from build123d import *

# Parameters (mm, degrees)
BOSS_EXTRUDE1_DEPTH  = 90
SKETCH2_W            = 30
SKETCH2_H            = 40
CUT_EXTRUDE1_DEPTH   = 90
SKETCH3_W            = 20
SKETCH3_H            = 20
CUT_EXTRUDE2_DEPTH   = 90
SKETCH4_W            = 80
SKETCH4_H            = 20
CUT_EXTRUDE3_DEPTH   = 90
SKETCH5_W            = 30
SKETCH5_H            = 30
CUT_EXTRUDE4_DEPTH   = 90
CUT_EXTRUDE6_DEPTH   = 40
BOSS_EXTRUDE6_DEPTH  = 30
CUT_EXTRUDE7_DEPTH   = 20
SKETCH12_W           = 10
SKETCH12_H           = 30
CUT_EXTRUDE8_DEPTH   = 20
SKETCH13_W           = 20
SKETCH13_H           = 30
CUT_EXTRUDE9_DEPTH   = 20
SKETCH14_W           = 21.421822341
SKETCH14_H           = 40
BOSS_EXTRUDE7_DEPTH  = 10
SKETCH16_W           = 20
SKETCH16_H           = 60
BOSS_EXTRUDE8_DEPTH  = 30
SKETCH17_W           = 30
SKETCH17_H           = 30
CUT_EXTRUDE10_DEPTH  = 20
SKETCH18_W           = 90
SKETCH18_H           = 30
BOSS_EXTRUDE9_DEPTH  = 10
SKETCH19_W           = 90
SKETCH19_H           = 20
BOSS_EXTRUDE10_DEPTH = 20
SKETCH21_W           = 10.0001
SKETCH21_H           = 30
BOSS_EXTRUDE13_DEPTH = 30
SKETCH22_W           = 10
SKETCH22_H           = 30
CUT_EXTRUDE13_DEPTH  = 29.999
SKETCH23_W           = 30
SKETCH23_H           = 29.999
CUT_EXTRUDE14_DEPTH  = 1
SKETCH24_W           = 10.0001
SKETCH24_H           = 30
CUT_EXTRUDE15_DEPTH  = 1
SKETCH25_W           = 10
SKETCH25_H           = 30
CUT_EXTRUDE16_DEPTH  = 10
SKETCH27_W           = 10
SKETCH27_H           = 10
CUT_EXTRUDE18_DEPTH  = 30
SKETCH30_W           = 20
SKETCH30_H           = 20
BOSS_EXTRUDE16_DEPTH = 30
SKETCH31_W           = 30
SKETCH31_H           = 20
BOSS_EXTRUDE17_DEPTH = 10


with BuildPart() as part:
    # Sketch1 → Boss-Extrude1 (new body)
    with BuildSketch(Plane.XY):
        with BuildLine():
            ThreePointArc((0, -40), (40, 0), (0, 40))
            Line((0, 40), (0, 20))
            ThreePointArc((0, 20), (14.142135624, 14.142135624), (20, 0))
            ThreePointArc((20, 0), (0, -20), (-20, 0))
            Line((-20, 0), (-40, 0))
            ThreePointArc((-40, 0), (-28.284271247, -28.284271247), (0, -40))
        make_face()
        with BuildLine():
            Line((70, 40), (0, 40))
            ThreePointArc((0, 40), (40, 0), (0, -40))
            Line((0, -40), (70, -40))
            Line((70, -40), (70, 40))
        make_face()
    extrude(amount=BOSS_EXTRUDE1_DEPTH)

    # Sketch2 → Cut-Extrude1 (cut)
    with BuildSketch(Plane.XY.offset(90)):
        with Locations((55, 0)):
            Rectangle(SKETCH2_W, SKETCH2_H)
    extrude(amount=-CUT_EXTRUDE1_DEPTH, mode=Mode.SUBTRACT)

    # Sketch3 → Cut-Extrude2 (cut)
    with BuildSketch(Plane.XY.offset(90)):
        with Locations((60, 30)):
            Rectangle(SKETCH3_W, SKETCH3_H)
    extrude(amount=-CUT_EXTRUDE2_DEPTH, mode=Mode.SUBTRACT)

    # Sketch4 → Cut-Extrude3 (cut)
    with BuildSketch(Plane(origin=(0, -40, 0), x_dir=(1, 0, 0), z_dir=(0, 1, 0))):
        with Locations((0, -80)):
            Rectangle(SKETCH4_W, SKETCH4_H)
    extrude(amount=CUT_EXTRUDE3_DEPTH, mode=Mode.SUBTRACT)

    # Sketch5 → Cut-Extrude4 (cut)
    with BuildSketch(Plane(origin=(0, 0, 0), x_dir=(0, 0, -1), z_dir=(1, 0, 0))):
        with Locations((-85, 25)):
            Rectangle(SKETCH5_W, SKETCH5_H)
    extrude(amount=CUT_EXTRUDE4_DEPTH, mode=Mode.SUBTRACT)

    # Sketch7 → Cut-Extrude6 (cut)
    with BuildSketch(Plane.XY.offset(70)):
        with BuildLine():
            Line((20, 0), (40, 0))
            Line((40, 0), (40, 40))
            Line((40, 40), (0, 40))
            Line((0, 40), (0, 20))
            ThreePointArc((0, 20), (14.142135624, 14.142135624), (20, 0))
        make_face()
    extrude(amount=-CUT_EXTRUDE6_DEPTH, mode=Mode.SUBTRACT)

    # Sketch10 → Boss-Extrude6 (add)
    with BuildSketch(Plane(origin=(70, 0, 0), x_dir=(0, 0, -1), z_dir=(1, 0, 0))):
        Polygon((-70, 20), (-70, 10), (-90, 10), (-90, -20), (-37.089362558, -20), (-21.421822341, -20), (-21.421822341, 20), align=None)
    extrude(amount=-BOSS_EXTRUDE6_DEPTH)

    # Sketch11 → Cut-Extrude7 (cut)
    with BuildSketch(Plane(origin=(70, 0, 0), x_dir=(0, 0, -1), z_dir=(1, 0, 0))):
        Polygon((-21.421822341, -20), (-70, -20), (-70, 10), (-70, 20), (-21.421822341, 20), align=None)
    extrude(amount=-CUT_EXTRUDE7_DEPTH, mode=Mode.SUBTRACT)

    # Sketch12 → Cut-Extrude8 (cut)
    with BuildSketch(Plane(origin=(50, 0, 0), x_dir=(0, 0, -1), z_dir=(1, 0, 0))):
        with Locations((-65, 25)):
            Rectangle(SKETCH12_W, SKETCH12_H)
    extrude(amount=-CUT_EXTRUDE8_DEPTH, mode=Mode.SUBTRACT)

    # Sketch13 → Cut-Extrude9 (cut)
    with BuildSketch(Plane(origin=(0, 0, 70), x_dir=(-1, 0, 0), z_dir=(0, 0, -1))):
        with Locations((-60, -5)):
            Rectangle(SKETCH13_W, SKETCH13_H)
    extrude(amount=-CUT_EXTRUDE9_DEPTH, mode=Mode.SUBTRACT)

    # Sketch14 → Boss-Extrude7 (add)
    with BuildSketch(Plane(origin=(40, 0, 0), x_dir=(0, 0, -1), z_dir=(1, 0, 0))):
        with Locations((-10.710911171, 0)):
            Rectangle(SKETCH14_W, SKETCH14_H)
    extrude(amount=BOSS_EXTRUDE7_DEPTH)

    # Sketch16 → Boss-Extrude8 (add)
    with BuildSketch(Plane(origin=(0, 40, 0), x_dir=(1, 0, 0), z_dir=(0, 1, 0))):
        with Locations((60, -30)):
            Rectangle(SKETCH16_W, SKETCH16_H)
    extrude(amount=-BOSS_EXTRUDE8_DEPTH)

    # Sketch17 → Cut-Extrude10 (cut)
    with BuildSketch(Plane(origin=(70, 0, 0), x_dir=(0, 0, -1), z_dir=(1, 0, 0))):
        with Locations((-15, 25)):
            Rectangle(SKETCH17_W, SKETCH17_H)
    extrude(amount=-CUT_EXTRUDE10_DEPTH, mode=Mode.SUBTRACT)

    # Sketch18 → Boss-Extrude9 (add)
    with BuildSketch(Plane(origin=(50, 0, 0), x_dir=(0, 0, -1), z_dir=(1, 0, 0))):
        with Locations((-45, -5)):
            Rectangle(SKETCH18_W, SKETCH18_H)
    extrude(amount=BOSS_EXTRUDE9_DEPTH)

    # Sketch19 → Boss-Extrude10 (add)
    with BuildSketch(Plane(origin=(70, 0, 0), x_dir=(0, 0, -1), z_dir=(1, 0, 0))):
        with Locations((-45, -30)):
            Rectangle(SKETCH19_W, SKETCH19_H)
    extrude(amount=BOSS_EXTRUDE10_DEPTH)

    # Sketch21 → Boss-Extrude13 (add)
    with BuildSketch(Plane(origin=(0, 0, 30), x_dir=(-1, 0, 0), z_dir=(0, 0, -1))):
        with Locations((-64.99995, 25)):
            Rectangle(SKETCH21_W, SKETCH21_H)
    extrude(amount=BOSS_EXTRUDE13_DEPTH)

    # Sketch22 → Cut-Extrude13 (cut)
    with BuildSketch(Plane.XZ.offset(-10)):
        with Locations((65, 15)):
            Rectangle(SKETCH22_W, SKETCH22_H)
    extrude(amount=-CUT_EXTRUDE13_DEPTH, mode=Mode.SUBTRACT)

    # Sketch23 → Cut-Extrude14 (cut)
    with BuildSketch(Plane(origin=(60, 0, 0), x_dir=(0, 0, -1), z_dir=(1, 0, 0))):
        with Locations((-15, 24.9995)):
            Rectangle(SKETCH23_W, SKETCH23_H)
    extrude(amount=-CUT_EXTRUDE14_DEPTH, mode=Mode.SUBTRACT)

    # Sketch24 → Cut-Extrude15 (cut)
    with BuildSketch(Plane.XZ.offset(-39.999)):
        with Locations((64.99995, 15)):
            Rectangle(SKETCH24_W, SKETCH24_H)
    extrude(amount=-CUT_EXTRUDE15_DEPTH, mode=Mode.SUBTRACT)

    # Sketch25 → Cut-Extrude16 (cut)
    with BuildSketch(Plane(origin=(0, 10, 0), x_dir=(1, 0, 0), z_dir=(0, 1, 0))):
        with Locations((55, -15)):
            Rectangle(SKETCH25_W, SKETCH25_H)
    extrude(amount=-CUT_EXTRUDE16_DEPTH, mode=Mode.SUBTRACT)

    # Sketch27 → Cut-Extrude18 (cut)
    with BuildSketch(Plane.XY.offset(60)):
        with Locations((65, 15)):
            Rectangle(SKETCH27_W, SKETCH27_H)
    extrude(amount=-CUT_EXTRUDE18_DEPTH, mode=Mode.SUBTRACT)

    # Sketch30 → Boss-Extrude16 (add)
    with BuildSketch(Plane(origin=(0, 0, 30), x_dir=(-1, 0, 0), z_dir=(0, 0, -1))):
        with Locations((-60, 30)):
            Rectangle(SKETCH30_W, SKETCH30_H)
    extrude(amount=BOSS_EXTRUDE16_DEPTH)

    # Sketch31 → Boss-Extrude17 (add)
    with BuildSketch(Plane(origin=(50, 0, 0), x_dir=(0, 0, -1), z_dir=(1, 0, 0))):
        with Locations((-15, 10)):
            Rectangle(SKETCH31_W, SKETCH31_H)
    extrude(amount=BOSS_EXTRUDE17_DEPTH)


solid = part.part
Geometry: final body of the model. Coordinates: model frame, mm. A direction names the side the tool comes from. Round coordinates to 2 decimals unless told otherwise and drop trailing zeros. Write each loop counter-clockwise with the first axis right and the second up, starting at its lowest first coordinate (ties: lowest second). Pieces come first, ordered by that corner, then holes. Notation, with made-up numbers: M -18,23 L -5,23 A12 ccw -5,37 Z; hole C -15,19 d9. An arc over 180 degrees is marked long. Write item = value, one per line.
Item 1: Material intervals for line 1 along X through (y, z) = (4.5, 31); line 2 along Y through (x, z) = (70, 85.5); line 3 along Z through (x, y) = (13, 32.5), sorted ascending. Write a range as [from, to].
Findings:
line_1 = [40, 60]
line_2 = [-40, -20]
line_3 = [0, 30]
Item 2: Section query C-C on x = 7. Return loops of the section in (y, z) (3 decimals).
Findings:
outline = M -40,0 L -18.735,0 L -18.735,70 L -40,70 Z; M 18.735,0 L 40,0 L 40,30 L 18.735,30 Z
Item 3: Pull-direction query (Y, two-part tool) for faces 1 (the face through (30, 0, 50)), 2 (the face through (65, 20, 30)), 3 (the face through (59, -21, 90)), 4 (the face through (-28.594, -27.972, 34.51)); classes: pulls with the +Y half, pulls with the -Y half, needs draft (parallel to the pull), parting line crosses it, or undercut.
Findings:
face_1 = pulls with the +Y half
face_2 = undercut
face_3 = needs draft
face_4 = pulls with the -Y half
Item 4: Section query B-B on z = 7. Return loops of the section in (x, y).
Findings:
outline = M -40,0 A40 ccw 0,-40 L 90,-40 L 90,-20 L 60,-20 L 60,20 L 70,20 L 70,40 L 0,40 L 0,20 A20 cw long -20,0 Z
Item 5: Section query D-D on y = 35.5. Return loops of the section in (x, z).
Findings:
outline = M 0,0 L 70,0 L 70,60 L 40,60 L 40,30 L 0,30 Z
Item 6: Access query for faces 5 (the face through (60, 0, 46)), 6 (the face through (70, 30, 30)), 7 (the face through (55, 25, 60)), 8 (the face through (-0.6, -20.3, 70)). Directions: +Z, -Z, +X, -X, +Y, -Y. A direction counts if a zero-diameter tool reaches every point of the face in a straight line with its end or side. Return the directions, or none.
Findings:
face_5 = +Z, -Z, +X
face_6 = +Z, -Z, +X, +Y
face_7 = +Z, +X, -X, +Y
face_8 = +Z, -X, +Y, -Y
Item 7: Pin query (flat end, axial travel): P1, Ø20, axis at x = 28, y = 17.5, coming from the +Z side; P2, Ø6, axis at y = -14, z = 47, coming from the -X side; P3, Ø5, axis at x = 26.5, y = -0.5, coming from the +Z side; P4, Ø6, axis at x = 14.5, y = -19, coming from the -Z side. Return the tip coordinate at first contact, or that it passes through.
Findings:
P1 = 30
P2 = -38.46
P3 = 70
P4 = 0
Item 8: Section query A-A on y = -4. Return loops of the section in (x, z).
Findings:
outline = M -39.8,0 L -19.6,0 L -19.6,70 L -39.8,70 Z; M 19.6,0 L 60,0 L 60,90 L 40,90 L 40,70 L 19.6,70 Z
